Build history of the part. All positions in model axes, mm. Face numbers are marked on the shaded views. A direction names the side the tool comes from. Coordinates: 2 decimals unless noted, no trailing zeros. Loops run counter-clockwise (first coordinate to the right, second up) from the corner with the lowest first, then second, coordinate; pieces in that order, holes last. Notation, with made-up numbers: (89, 14) - (123, 14) arc R24 ccw to (123, 45) - close; hole circle Ø3 at (56, 77.5). An arc over 180 degrees is marked (long way). One line per item, written item: value.
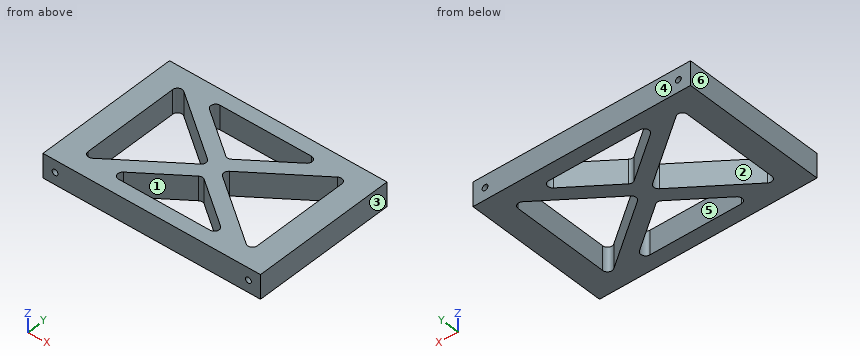
```python
from build123d import *

# Parameters (mm, degrees)
SKIZZE1_W                       = 90
SKIZZE1_H                       = 60
AUFSATZ_LINEAR_AUSTRAGEN1_DEPTH = 10
SCHNITT_LINEAR_AUSTRAGEN1_DEPTH = 10
SKIZZE3_R                       = 1.2
SCHNITT_LINEAR_AUSTRAGEN2_DEPTH = 84


with BuildPart() as part:
    # Skizze1 → Aufsatz-Linear austragen1 (new body)
    with BuildSketch(Plane.XY):
        with Locations((45, 30)):
            Rectangle(SKIZZE1_W, SKIZZE1_H)
    extrude(amount=AUFSATZ_LINEAR_AUSTRAGEN1_DEPTH)

    # Skizze2 → Schnitt-Linear austragen1 (cut)
    with BuildSketch(Plane.XY.offset(10)):
        with BuildLine():
            Line((10, 50.05034464), (10, 9.94965536))
            ThreePointArc((10, 9.94965536), (11.096486968, 8.165372815), (13.183664201, 8.337532828))
            Line((13.183664201, 8.337532828), (40.491757454, 28.387877468))
            ThreePointArc((40.491757454, 28.387877468), (41.308093253, 30), (40.491757454, 31.612122532))
            Line((40.491757454, 31.612122532), (13.183664201, 51.662467172))
            ThreePointArc((13.183664201, 51.662467172), (11.096486968, 51.834627185), (10, 50.05034464))
        make_face()
        with BuildLine():
            Line((43.816335799, 36.499330073), (24.900464067, 50.387877468))
            ThreePointArc((24.900464067, 50.387877468), (24.183569789, 52.622798095), (26.084128268, 54))
            Line((26.084128268, 54), (63.915871732, 54))
            ThreePointArc((63.915871732, 54), (65.816430211, 52.622798095), (65.099535933, 50.387877468))
            Line((65.099535933, 50.387877468), (46.183664201, 36.499330073))
            ThreePointArc((46.183664201, 36.499330073), (45, 36.111452606), (43.816335799, 36.499330073))
        make_face()
        with BuildLine():
            Line((26.084128268, 6), (63.915871732, 6))
            ThreePointArc((63.915871732, 6), (65.816430211, 7.377201905), (65.099535933, 9.612122532))
            Line((65.099535933, 9.612122532), (46.183664201, 23.500669927))
            ThreePointArc((46.183664201, 23.500669927), (45, 23.888547394), (43.816335799, 23.500669927))
            Line((43.816335799, 23.500669927), (24.900464067, 9.612122532))
            ThreePointArc((24.900464067, 9.612122532), (24.183569789, 7.377201905), (26.084128268, 6))
        make_face()
        with BuildLine():
            Line((80, 50.05034464), (80, 9.94965536))
            ThreePointArc((80, 9.94965536), (78.903513032, 8.165372815), (76.816335799, 8.337532828))
            Line((76.816335799, 8.337532828), (49.508242546, 28.387877468))
            ThreePointArc((49.508242546, 28.387877468), (48.691906747, 30), (49.508242546, 31.612122532))
            Line((49.508242546, 31.612122532), (76.816335799, 51.662467172))
            ThreePointArc((76.816335799, 51.662467172), (78.903513032, 51.834627185), (80, 50.05034464))
        make_face()
    extrude(amount=-SCHNITT_LINEAR_AUSTRAGEN1_DEPTH, mode=Mode.SUBTRACT)

    # Skizze3 → Schnitt-Linear austragen2 (cut)
    with BuildSketch(Plane(origin=(0, 60, 0), x_dir=(1, 0, 0), z_dir=(0, 1, 0))):
        with Locations(Location((5, -5, 0), (0, 0, 270))):
            Circle(SKIZZE3_R)
        with Locations(Location((85, -5, 0), (0, 0, 270))):
            Circle(SKIZZE3_R)
    extrude(amount=-SCHNITT_LINEAR_AUSTRAGEN2_DEPTH, mode=Mode.SUBTRACT)


solid = part.part
```
Item 1: Tool access for the marked faces 5 and 6: list every direction of +Z, -Z, +X, -X, +Y, -Y with a clear straight run to the whole face (end or side of a thin tool).
Check result:
face 5: +Z, -Z
face 6: +Z, -Z, -X, +Y, -Y
Item 2: Cut at B-B, the plane y = 26. Write the cut outline in (x, z).
Check result:
outline: (0, 0) - (10, 0) - (10, 10) - (0, 10) - close; (37.24, 0) - (52.76, 0) - (52.76, 10) - (37.24, 10) - close; (80, 0) - (90, 0) - (90, 10) - (80, 10) - close; hole circle Ø2.4 at (5, 5); hole circle Ø2.4 at (85, 5)
Item 3: Cut at C-C, the plane y = 48.5. Write the cut outline in (x, z), then the cut area to 3 significant figures.
Check result:
outline: (0, 0) - (10, 0) - (10, 10) - (0, 10) - close; (17.49, 0) - (27.47, 0) - (27.47, 10) - (17.49, 10) - close; (62.53, 0) - (72.51, 0) - (72.51, 10) - (62.53, 10) - close; (80, 0) - (90, 0) - (90, 10) - (80, 10) - close; hole circle Ø2.4 at (5, 5); hole circle Ø2.4 at (85, 5)
area: 391 mm^2
Item 4: Cut at D-D, the plane z = 5. Give the number of separate pieces and of enclosed holes in the cut face, then the cut area to 3 significant figures.
Check result:
separate pieces: 3
enclosed holes: 4
area: 2,670 mm^2
Item 5: Probe probe 1 along X at (y, z) = (30, 5); probe 2 along Y at (x, z) = (12, 3.75); probe 3 along X at (y, z) = (30, 3.5). List the from-to ranges inside material, lowest first. Write a range as from..to.
Check result:
probe 1: x = 0..3.8, 6.2..10, 41.31..48.69, 80..83.8, 86.2..90
probe 2: y = 0..7.95, 52.05..60
probe 3: x = 0..10, 41.31..48.69, 80..90
Item 6: Cut at A-A, the plane x = 85. Write the cut outline in (y, z), then the cut area to 3 significant figures.
Check result:
outline: (0, 0) - (60, 0) - (60, 3.8) - (0, 3.8) - close; (0, 6.2) - (60, 6.2) - (60, 10) - (0, 10) - close
area: 456 mm^2
Item 7: Pull direction Y, two halves, no side cores. Call the marked faces 1, 2, 3 and 4: released by +Y, released by -Y, zero draft, split by the parting line, or undercut.
Check result:
face 1: undercut
face 2: undercut
face 3: zero draft
face 4: released by +Y
